Build history of the part. All positions in model axes, mm. Face numbers are marked on the shaded views. A direction names the side the tool comes from. Coordinates: 2 decimals unless noted, no trailing zeros. Loops run counter-clockwise (first coordinate to the right, second up) from the corner with the lowest first, then second, coordinate; pieces in that order, holes last.
(1) Tool access for the marked faces 3, 4 and 5: list every direction of +Z, -Z, +X, -X, +Y, -Y with a clear straight run to the whole face (end or side of a thin tool).
(2) Two-plate mould, pull along X, no slides. Class the marked faces 1 and 2: pulls with the +X half, pulls with the -X half, needs draft (parallel to the pull), parting line crosses it, or undercut.
(3) Flat gauge pins, fed straight in: P1, Ø6, axis at x = -9.5, y = 33, coming from the +Z side; P2, Ø3, axis at x = -2.5, z = 2.5, coming from the -Y side; P3, Ø8, axis at x = 14.5, z = 7, coming from the +Y side. Where does each tip first touch, or does it go through?
(4) Slice it at C-C (z = 9.25). Give the cut face in (x, y).
(5) Wall check: L1, parallel to Z at x = -21, y = -11; L2, parallel to X at y = -36, z = 6; L3, parallel to X at y = -33, z = 6.75. Give the ranges that are in metal, low to high.
(6) Slice it at B-B (x = 0). Give the cut face in (y, z), and give its area (3 significant figures).
(7) Slice it at A-A (y = 0). Give the cut face in (x, z), and give its area (3 significant figures).
from build123d import *

# Parameters (mm, degrees)
F3_DEPTH      = 126
F3_DEPTH_BACK = 15.401


# Not quite as in the source:
# - an extrude ends at something that could not be found from the text; its depth is read off the source's solid


with BuildPart() as f1:
    # F0 (on Front) → F1 (revolve)
    with BuildSketch(Plane.XZ):
        with BuildLine():
            Line((0, 0), (38.1, 0))
            Line((38.1, 0), (38.1, 4.4))
            Line((38.1, 4.4), (42.5, 4.4))
            Line((42.5, 4.4), (42.5, 5.4))
            ThreePointArc((42.5, 5.4), (41.9142135624, 6.8142135624), (40.5, 7.4))
            Line((40.5, 7.4), (13.608495283, 7.4))
            ThreePointArc((13.608495283, 7.4), (11.8592103205, 8.4304629352), (11.912498675, 10.45999788))
            Line((11.912498675, 10.45999788), (13.087501325, 12.34000212))
            ThreePointArc((13.087501325, 12.34000212), (13.1407896795, 14.3695370648), (11.391504717, 15.4))
            Line((11.391504717, 15.4), (0, 15.4))
            Line((0, 15.4), (0, 0))
        make_face()
    revolve(axis=Axis((0, 0, 11.4377464585), (0, 0, -1)))

    # F2 (on Top) → F3 (cut, two sides)
    with BuildSketch(Plane.XY) as f3_sk:
        with BuildLine():
            ThreePointArc((5, -33.1), (0, -28.1), (-5, -33.1))
            Line((-5, -33.1), (-5, -42.5))
            Line((-5, -42.5), (5, -42.5))
            Line((5, -42.5), (5, -33.1))
        make_face()
    extrude(amount=-F3_DEPTH, mode=Mode.SUBTRACT)
    extrude(f3_sk.sketch, amount=F3_DEPTH_BACK, mode=Mode.SUBTRACT)


solid = f1.part
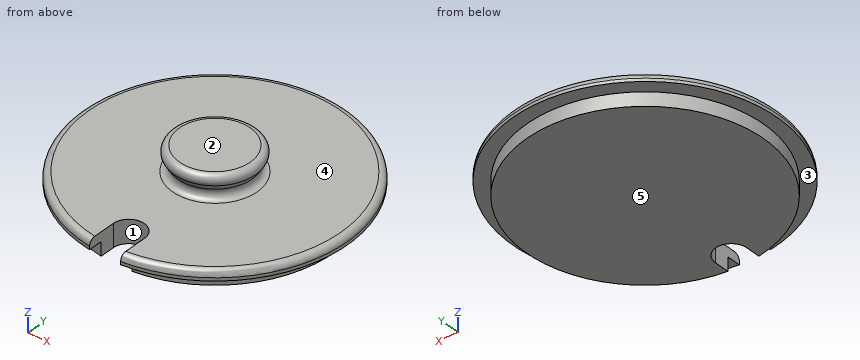
Response values:
1. face 3: -Z
1. face 4: +Z
1. face 5: -Z, +X, -X, +Y, -Y
2. face 1: undercut
2. face 2: needs draft
3. P1: stops at z = 7.4
3. P2: stops at y = -30.1
3. P3: stops at y = 41.11
4. outline: circle Ø23.23 at (0, 0)
5. L1: z = 0 to 7.4
5. L2: x = -22.41 to -5, 5 to 22.41
5. L3: x = -25.94 to -5, 5 to 25.94
6. outline: (-28.1, 0) - (38.1, 0) - (38.1, 4.4) - (42.5, 4.4) - (42.5, 5.4) arc R2 ccw to (40.5, 7.4) - (13.61, 7.4) arc R2 cw to (11.91, 10.46) - (13.09, 12.34) arc R2 ccw to (11.39, 15.4) - (-11.39, 15.4) arc R2 ccw to (-13.09, 12.34) - (-11.91, 10.46) arc R2 cw to (-13.61, 7.4) - (-28.1, 7.4) - close
6. area: 702 mm2
7. outline: (-42.5, 4.4) - (-38.1, 4.4) - (-38.1, 0) - (38.1, 0) - (38.1, 4.4) - (42.5, 4.4) - (42.5, 5.4) arc R2 ccw to (40.5, 7.4) - (13.61, 7.4) arc R2 cw to (11.91, 10.46) - (13.09, 12.34) arc R2 ccw to (11.39, 15.4) - (-11.39, 15.4) arc R2 ccw to (-13.09, 12.34) - (-11.91, 10.46) arc R2 cw to (-13.61, 7.4) - (-40.5, 7.4) arc R2 ccw to (-42.5, 5.4) - close
7. area: 789 mm2
